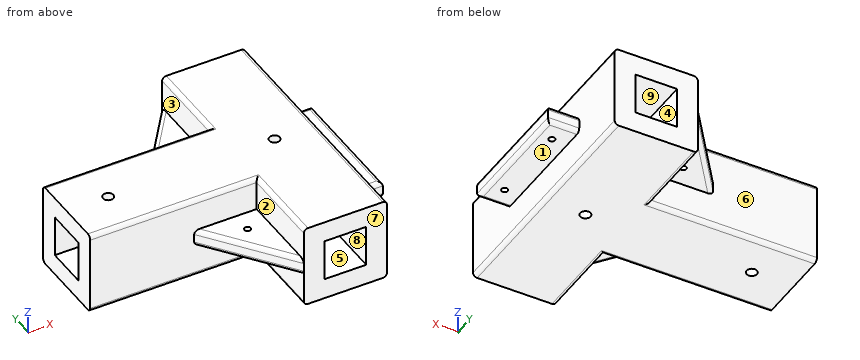
```python
from build123d import *

# Parameters (mm, degrees)
SKETCH1_W                = 40
SKETCH1_H                = 40
SKETCH1_W_2              = 20
SKETCH1_H_2              = 20
BOSS_EXTRUDE1_DEPTH      = 120
SKETCH2_W                = 40
SKETCH2_H                = 40
SKETCH2_W_2              = 20
SKETCH2_H_2              = 20
BOSS_EXTRUDE2_DEPTH      = 80
BOSS_EXTRUDE3_DEPTH      = 4
BOSS_EXTRUDE3_DEPTH_BACK = 4
SKETCH5_R                = 1.5
SKETCH5_W                = 15
SKETCH5_H                = 60
SKETCH7_W                = 20
SKETCH7_H                = 20
CUT_EXTRUDE2_DEPTH       = 30
SKETCH8_R                = 2.5
CUT_EXTRUDE3_DEPTH       = 150.666295471
FILLET1_R                = 2
FILLET2_R                = 2
FILLET3_R                = 2
FILLET4_R                = 2
FILLET5_R                = 2


with BuildPart() as part:
    # Sketch1 → Boss-Extrude1 (new body)
    with BuildSketch(Plane(origin=(0, 0, 0), x_dir=(1, 0, 0), z_dir=(0, 1, 0))):
        with Locations((20, 20)):
            Rectangle(SKETCH1_W, SKETCH1_H)
        with Locations((20, 20)):
            Rectangle(SKETCH1_W_2, SKETCH1_H_2, mode=Mode.SUBTRACT)
    extrude(amount=BOSS_EXTRUDE1_DEPTH)

    # Sketch2 → Boss-Extrude2 (add)
    with BuildSketch(Plane.ZY):
        with Locations((-20, 60)):
            Rectangle(SKETCH2_W, SKETCH2_H)
        with Locations((-20, 60)):
            Rectangle(SKETCH2_W_2, SKETCH2_H_2, mode=Mode.SUBTRACT)
    extrude(amount=BOSS_EXTRUDE2_DEPTH)

    # Sketch5 → Boss-Extrude3 (add, two sides: drawn at the far end of the back side and taken through both)
    # profile 1 of 3: a face of its own
    with BuildSketch(Plane.XY.offset(-20).offset(-BOSS_EXTRUDE3_DEPTH_BACK)):
        Polygon((0, 120), (0, 80), (-30, 80), align=None)
        with Locations((-10, 90)):
            Circle(SKETCH5_R, mode=Mode.SUBTRACT)
    # profile 2 of 3: a face of its own
    with BuildSketch(Plane.XY.offset(-20).offset(-BOSS_EXTRUDE3_DEPTH_BACK)):
        Polygon((0, 0), (-30, 40), (0, 40), align=None)
        with Locations((-10, 30)):
            Circle(SKETCH5_R, mode=Mode.SUBTRACT)
    # profile 3 of 3: a face of its own
    with BuildSketch(Plane.XY.offset(-20).offset(-BOSS_EXTRUDE3_DEPTH_BACK)):
        with Locations((47.5, 60)):
            Rectangle(SKETCH5_W, SKETCH5_H)
        with Locations((47.5, 80)):
            Circle(SKETCH5_R, mode=Mode.SUBTRACT)
        with Locations((47.5, 40)):
            Circle(SKETCH5_R, mode=Mode.SUBTRACT)
    extrude(amount=BOSS_EXTRUDE3_DEPTH + BOSS_EXTRUDE3_DEPTH_BACK)

    # Sketch7 → Cut-Extrude2 (cut)
    with BuildSketch(Plane.ZY):
        with Locations((-20, 60)):
            Rectangle(SKETCH7_W, SKETCH7_H)
    extrude(amount=-CUT_EXTRUDE2_DEPTH, mode=Mode.SUBTRACT)

    # Sketch8 → Cut-Extrude3 (cut, through all)
    with BuildSketch(Plane.XY):
        with Locations((-60, 60)):
            Circle(SKETCH8_R)
        with Locations((20, 60)):
            Circle(SKETCH8_R)
    extrude(amount=-CUT_EXTRUDE3_DEPTH, mode=Mode.SUBTRACT)

    # Fillet1
    fillet1_edges = [part.edges().sort_by_distance(p)[0] for p in [
        (-40, 80, 0),
    ]]
    fillet(fillet1_edges, radius=FILLET1_R)

    # Fillet2
    fillet2_edges = [part.edges().sort_by_distance(p)[0] for p in [
        (-40, 80, -40),
        (-40, 40, -40),
        (-40, 40, 0),
    ]]
    fillet(fillet2_edges, radius=FILLET2_R)

    # Fillet3
    fillet3_edges = [part.edges().sort_by_distance(p)[0] for p in [
        (40, 60, -40),
        (40, 60, 0),
        (0, 21, -40),
        (0, 21, 0),
        (0, 99, -40),
        (0, 99, 0),
    ]]
    fillet(fillet3_edges, radius=FILLET3_R)

    # Fillet4
    fillet4_edges = [part.edges().sort_by_distance(p)[0] for p in [
        (47.5, 90, -24),
        (55, 60, -24),
        (47.5, 30, -24),
        (47.5, 30, -16),
        (55, 60, -16),
        (47.5, 90, -16),
    ]]
    fillet(fillet4_edges, radius=FILLET4_R)

    # Fillet5
    fillet5_edges = [part.edges().sort_by_distance(p)[0] for p in [
        (-15, 20, -24),
        (-15, 20, -16),
        (-15, 100, -24),
        (-15, 100, -16),
    ]]
    fillet(fillet5_edges, radius=FILLET5_R)


solid = part.part
```
Source: CAD feature listing. Evaluate the final solid. Frame: model axes, mm. Face numbers are marked on the shaded views. A direction names the side the tool comes from. Give positions to 0.01 mm unless a question says otherwise; leave off trailing zeros. Loops run counter-clockwise (first coordinate to the right, second up) from the corner with the lowest first, then second, coordinate; pieces in that order, holes last. Notation, with made-up numbers: (60, 22.5) -> (110, 22.5) arc R11 cw to (110, 35.5) -> close; hole circle Ø4 at (88, 87). An arc over 180 degrees is marked (long way). Use a Markdown table: item, result. Add a question column.
(1) Access query for the marked faces 1, 2, 3, 4 and 5. Directions: +Z, -Z, +X, -X, +Y, -Y. A direction counts if a zero-diameter tool reaches every point of the face in a straight line with its end or side. Return the directions, or none.
(2) Section query D-D (z = -5). Output: boundary loops of the cut face in (x, y), then the cut area to 3 significant figures.
(3) Section query B-B (x = -60). Output: boundary loops of the cut face in (y, z), then the cut area to 3 significant figures.
(4) Ray query, line 1 (Y direction, x = -10, z = -18.5); line 2 (Z direction, x = -58.5, y = 57); line 3 (Y direction, x = -73.5, z = -29). Return the intervals inside material, ascending.
(5) Section query C-C (y = 60). Count the separate pieces of the cut face and the enclosed holes in it, then the cut area to 3 significant figures.
(6) Pull-direction query (Y, two-part tool) for the marked faces 6, 7, 8 and 9; classes: +Y half, -Y half, draft (parallel to the pull), parting line (faces both ways), or undercut.
(7) First-contact query: pin 1 Ø16 at (y, z) = (100.5, -20.5) entering from +X; pin 2 Ø6 at (y, z) = (13, -20.5) entering from -X; pin 3 Ø4.5 at (x, y) = (-60, 60) entering from -Z; pin 4 Ø2 at (x, z) = (-16.5, -28.5) entering from +Y. Flat tips, straight axial feed; report the tip coordinate or a pass-through.
(8) Section query A-A (z = -26.5). Output: boundary loops of the cut face in (x, y).
Checked values:
| question | item | result |
|---|---|---|
| 1 | face 1 | -Z, +X, +Y, -Y |
| 1 | face 2 | +Z, -X, -Y |
| 1 | face 3 | +Z, -X, +Y |
| 1 | face 4 | +Y, -Y |
| 1 | face 5 | none |
| 2 | outline | (-80, 40) -> (0, 40) -> (0, 0) -> (40, 0) -> (40, 120) -> (0, 120) -> (0, 80) -> (-80, 80) -> close; hole circle Ø5 at (-60, 60); hole circle Ø5 at (20, 60) |
| 2 | area | 7,960 mm^2 |
| 3 | outline | (40, -38) arc R2 ccw to (42, -40) -> (57.5, -40) -> (57.5, -30) -> (50, -30) -> (50, -10) -> (57.5, -10) -> (57.5, 0) -> (42, 0) arc R2 ccw to (40, -2) -> close; (62.5, -40) -> (78, -40) arc R2 ccw to (80, -38) -> (80, -2) arc R2 ccw to (78, 0) -> (62.5, 0) -> (62.5, -10) -> (70, -10) -> (70, -30) -> (62.5, -30) -> close |
| 3 | area | 1,100 mm^2 |
| 4 | line 1 | 13.33 to 28.5, 31.5 to 50, 70 to 88.5, 91.5 to 106.67 |
| 4 | line 2 | -40 to -30, -10 to 0 |
| 4 | line 3 | 40 to 50, 70 to 80 |
| 5 | separate pieces | 5 |
| 5 | enclosed holes | 0 |
| 5 | area | 2,520 mm^2 |
| 6 | face 6 | +Y half |
| 6 | face 7 | -Y half |
| 6 | face 8 | draft |
| 6 | face 9 | undercut |
| 7 | pin 1 | x = 40 |
| 7 | pin 2 | x = -12 |
| 7 | pin 3 | through |
| 7 | pin 4 | y = 80 |
| 8 | outline | (-80, 40) -> (0, 40) -> (0, 0) -> (10, 0) -> (10, 50) -> (-80, 50) -> close; (-80, 70) -> (10, 70) -> (10, 120) -> (0, 120) -> (0, 80) -> (-80, 80) -> close; (30, 0) -> (40, 0) -> (40, 120) -> (30, 120) -> close |
